The drawing under review shows one solid part. Ordinate dimensions are in mm from its lowest x, y, z. A direction names the side the tool comes from. Round coordinates to 2 decimals unless told otherwise and drop trailing zeros. Write each loop counter-clockwise with the first axis right and the second up, starting at its lowest first coordinate (ties: lowest second). Pieces come first, ordered by that corner, then holes.
Item 1: Machinability: for the marked faces 4, 5 and 6, which of the approach directions +Z, -Z, +X, -X, +Y, -Y give a long, thin tool a straight path to every point of the face, cutting with its end or side? Answer none if there is none.
Item 2: Draft analysis for pull direction Z (two halves, no side actions). For the marked faces 1, 2 and 3, state which applies: +Z half, -Z half, draft (parallel to the pull), parting line (faces both ways), or undercut.
Item 3: Add section B-B (x = 84.5). Give the boundary of the cut face in (y, z), plus the area to 3 significant figures.
Item 4: To check wall thickness, follow L1, parallel to Y at x = 7.5, z = 39; L2, parallel to X at y = 6.5, z = 9.5; L3, parallel to X at y = 15, z = 38. State the ranges of each line that lie inside material, in increasing order.
Item 5: Add section A-A (z = 46). Give the boundary of the cut face in (x, y).
Item 6: Clearance check with flat-ended pins moving along their axes: pin 1 Ø0.5 at (x, y) = (91.5, 10.5) entering from -Z; pin 2 Ø11 at (y, z) = (9, 48.5) entering from +X; pin 3 Ø5 at (x, y) = (77, 17) entering from -Z; pin 4 Ø8 at (x, z) = (83.5, 45.5) entering from +Y. State where each tip first meets the part, or that it passes through.
Item 7: Add section D-D (x = 47.5). Give the boundary of the cut face in (y, z), plus the area to 3 significant figures.
Item 8: Add section C-C (z = 13). Give the boundary of the cut face in (x, y), plus the area to 3 significant figures.
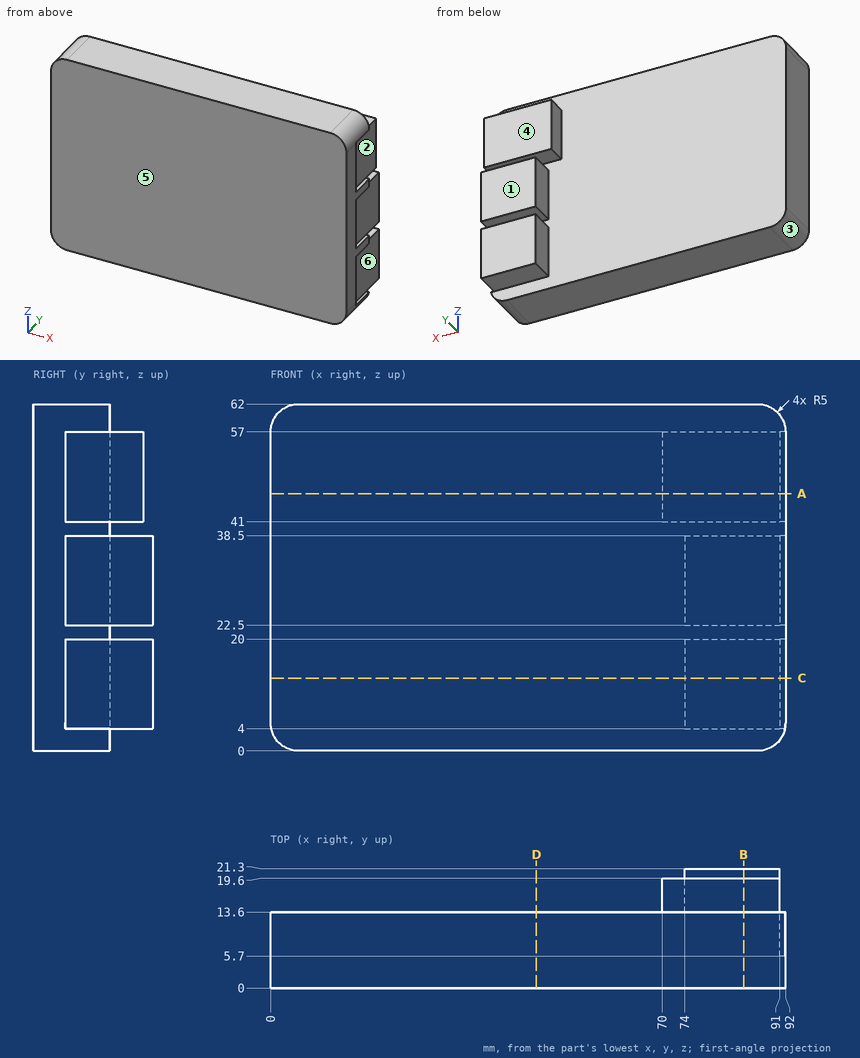
Numbers:
1. face 4: +Z, +X, -X, +Y
1. face 5: +Z, -Z, +X, -X, -Y
1. face 6: +X, +Y
2. face 1: draft
2. face 2: undercut
2. face 3: -Z half
3. outline: (0, 0) - (13.6, 0) - (13.6, 4) - (21.3, 4) - (21.3, 20) - (13.6, 20) - (13.6, 22.5) - (21.3, 22.5) - (21.3, 38.5) - (13.6, 38.5) - (13.6, 41) - (19.6, 41) - (19.6, 57) - (13.6, 57) - (13.6, 62) - (0, 62) - close
3. area: 1,190 mm2
4. L1: y = 0 to 13.6
4. L2: x = 0 to 91
4. L3: x = 74 to 91
5. outline: (0, 0) - (92, 0) - (92, 5.7) - (91, 5.7) - (91, 19.6) - (70, 19.6) - (70, 13.6) - (0, 13.6) - close
6. pin 1: stops at z = 2.37
6. pin 2: stops at x = 92
6. pin 3: stops at z = 4
6. pin 4: stops at y = 19.6
7. outline: (0, 0) - (13.6, 0) - (13.6, 62) - (0, 62) - close
7. area: 843 mm2
8. outline: (0, 0) - (92, 0) - (92, 5.7) - (91, 5.7) - (91, 21.3) - (74, 21.3) - (74, 13.6) - (0, 13.6) - close
8. area: 1,370 mm2
